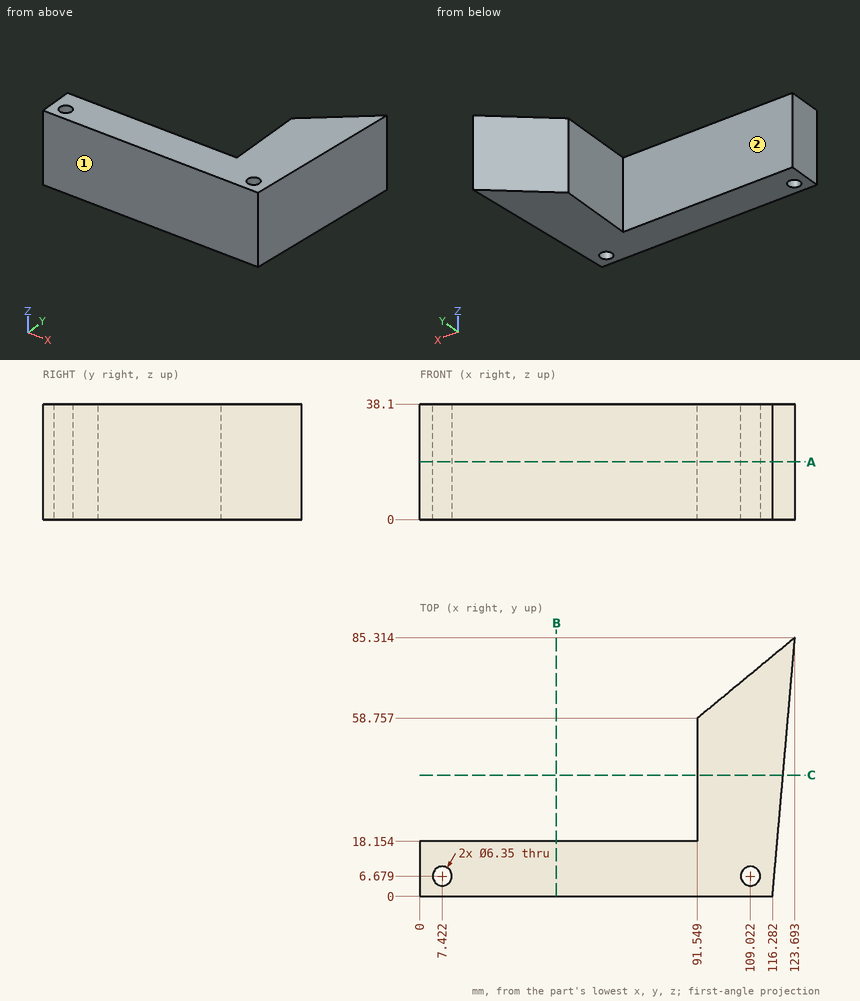
Source: three-view drawing plus pictorial views. Frame: mm from the lowest corner of the part. A direction names the side the tool comes from. Round coordinates to 2 decimals unless told otherwise and drop trailing zeros. Loops run counter-clockwise (first coordinate to the right, second up) from the corner with the lowest first, then second, coordinate; pieces in that order, holes last.
Q1. Ray query, line 1 (X direction, y = 4, z = 8.5) (1 decimal); line 2 (Y direction, x = 33, z = 7); line 3 (Y direction, x = 110, z = 15.5). Return the intervals inside material, ascending.
Q2. Section A-A, the plane z = 19. State how many separate pieces and enclosed holes the cut face has, plus the area to 3 significant figures.
Q3. Section B-B, the plane x = 45. Return loops of the section in (y, z), plus the area to 3 significant figures.
Q4. Access query for the marked faces 1 and 2. Directions: +Z, -Z, +X, -X, +Y, -Y. A direction counts if a zero-diameter tool reaches every point of the face in a straight line with its end or side. Return the directions, or none.
Q5. Section C-C, the plane y = 40. Return loops of the section in (x, z), plus the area to 3 significant figures.
Q6. First-contact query: P1, Ø2, axis at x = 95.5, z = 32, coming from the +Y side; P2, Ø10, axis at x = 109.02, y = 6.68, coming from the -Z side; P3, Ø1.5, axis at x = 103, z = 29, coming from the +Y side; P4, Ø1, axis at x = 66, z = 9, coming from the +Y side. Flat tips, straight axial feed; report the tip coordinate or a pass-through.
Solutions:
1. line 1: x = 0 to 5.7, 9.1 to 107.3, 110.7 to 116.6
1. line 2: y = 0 to 18.15
1. line 3: y = 0 to 3.66, 9.7 to 74
2. separate pieces: 1
2. enclosed holes: 2
2. area: 3,600 mm2
3. outline: (0, 0) - (18.15, 0) - (18.15, 38.1) - (0, 38.1) - close
3. area: 692 mm2
4. face 1: +Z, -Z, +X, -X, -Y
4. face 2: +Z, -Z, -X, +Y
5. outline: (91.55, 0) - (119.76, 0) - (119.76, 38.1) - (91.55, 38.1) - close
5. area: 1,070 mm2
6. P1: stops at y = 62.85
6. P2: stops at z = 0
6. P3: stops at y = 68.84
6. P4: stops at y = 18.15
